```python
from build123d import *

# Parameters (mm, degrees)
SKETCH1_R           = 0.425
SKETCH1_R_2         = 0.8
BOSS_EXTRUDE1_DEPTH = 1.6


with BuildPart() as part:
    # Sketch1 → Boss-Extrude1 (new body)
    with BuildSketch(Plane(origin=(0, 0, -0.0125), x_dir=(-1, 0, 0), z_dir=(0, 0, -1))):
        with BuildLine():
            Line((47.8, -40.8), (49.3, -40.8))
            Line((49.3, -40.8), (49.3, 39.2))
            Line((49.3, 39.2), (43.2, 45.3))
            Line((43.2, 45.3), (35.500000017, 45.3))
            Line((35.500000017, 45.3), (35.500000017, 43.8))
            ThreePointArc((35.500000017, 43.8), (35.207106799, 43.092893219), (34.500000017, 42.8))
            Line((34.500000017, 42.8), (4.500000014, 42.8))
            ThreePointArc((4.500000014, 42.8), (3.792893232, 43.092893219), (3.500000014, 43.8))
            Line((3.500000014, 43.8), (3.500000014, 45.3))
            Line((3.500000014, 45.3), (-43.2, 45.3))
            Line((-43.2, 45.3), (-49.3, 39.2))
            Line((-49.3, 39.2), (-49.3, -40.4))
            Line((-49.3, -40.4), (-47.8, -40.4))
            ThreePointArc((-47.8, -40.4), (-47.092893219, -40.692893219), (-46.8, -41.4))
            Line((-46.8, -41.4), (-46.8, -46))
            ThreePointArc((-46.8, -46), (-46.507106781, -46.707106781), (-45.8, -47))
            Line((-45.8, -47), (-36.3, -47))
            ThreePointArc((-36.3, -47), (-35.592893219, -47.292893219), (-35.3, -48))
            Line((-35.3, -48), (-35.3, -50))
            Line((-35.3, -50), (35.3, -50))
            Line((35.3, -50), (35.3, -48))
            ThreePointArc((35.3, -48), (35.592893219, -47.292893219), (36.3, -47))
            Line((36.3, -47), (45.8, -47))
            ThreePointArc((45.8, -47), (46.507106781, -46.707106781), (46.8, -46))
            Line((46.8, -46), (46.8, -41.8))
            ThreePointArc((46.8, -41.8), (47.092893219, -41.092893219), (47.8, -40.8))
        make_face()
        with Locations(Location((-13.87, 38.33, 0), (0, 0, 180))):
            Circle(SKETCH1_R, mode=Mode.SUBTRACT)
        with Locations(Location((-22.54, 39.6, 0), (0, 0, 180))):
            Circle(SKETCH1_R, mode=Mode.SUBTRACT)
        with Locations(Location((-23.81, 40.87, 0), (0, 0, 180))):
            Circle(SKETCH1_R, mode=Mode.SUBTRACT)
        with Locations(Location((-21.27, 40.87, 0), (0, 0, 180))):
            Circle(SKETCH1_R, mode=Mode.SUBTRACT)
        with Locations(Location((-13.87, 40.87, 0), (0, 0, 180))):
            Circle(SKETCH1_R, mode=Mode.SUBTRACT)
        with Locations(Location((-31.21, 40.87, 0), (0, 0, 180))):
            Circle(SKETCH1_R, mode=Mode.SUBTRACT)
        with Locations(Location((-16.41, 40.87, 0), (0, 0, 180))):
            Circle(SKETCH1_R, mode=Mode.SUBTRACT)
        with Locations(Location((-15.14, 39.6, 0), (0, 0, 180))):
            Circle(SKETCH1_R, mode=Mode.SUBTRACT)
        with Locations(Location((-29.94, 39.6, 0), (0, 0, 180))):
            Circle(SKETCH1_R, mode=Mode.SUBTRACT)
        with Locations(Location((-28.67, 40.87, 0), (0, 0, 180))):
            Circle(SKETCH1_R, mode=Mode.SUBTRACT)
        with Locations(Location((-28.67, 38.33, 0), (0, 0, 180))):
            Circle(SKETCH1_R, mode=Mode.SUBTRACT)
        with Locations(Location((-16.41, 38.33, 0), (0, 0, 180))):
            Circle(SKETCH1_R, mode=Mode.SUBTRACT)
        with Locations(Location((-21.27, 38.33, 0), (0, 0, 180))):
            Circle(SKETCH1_R, mode=Mode.SUBTRACT)
        with Locations(Location((-23.81, 38.33, 0), (0, 0, 180))):
            Circle(SKETCH1_R, mode=Mode.SUBTRACT)
        with Locations(Location((-31.21, 38.33, 0), (0, 0, 180))):
            Circle(SKETCH1_R, mode=Mode.SUBTRACT)
        with Locations((33.775, 38.54)):
            Circle(SKETCH1_R_2, mode=Mode.SUBTRACT)
        with Locations((5.225, 38.54)):
            Circle(SKETCH1_R_2, mode=Mode.SUBTRACT)
    extrude(amount=-BOSS_EXTRUDE1_DEPTH)


solid = part.part
```
The model under review builds one solid part; all positions refer to its coordinate system, in mm. Round coordinates to 2 decimals unless told otherwise and drop trailing zeros. Order: outer loops, then holes, each group sorted by start corner. A loop starts at its lowest first (then second) coordinate and runs counter-clockwise, first axis right, second up.
Item 1: To check wall thickness, follow probe 1 along Y at (x, z) = (21.27, 0.3) (3 decimals); probe 2 along Y at (x, z) = (15.14, 1) (3 decimals); probe 3 along Y at (x, z) = (-16, 0.5). State the ranges of each line that lie inside material, in increasing order.
Working result:
probe 1: y = -50 to 37.905, 38.755 to 40.445, 41.295 to 45.3
probe 2: y = -50 to 39.175, 40.025 to 45.3
probe 3: y = -50 to 42.8
Item 2: For pin 1 (0.5 mm diameter, centred on y = -48.5, z = 1, fed in from -X); pin 2 (0.5 mm diameter, centred on y = -44, z = 0.5, fed in from +X); pin 3 (0.8 mm diameter, centred on x = 48.5, z = 0.5, fed in from -Y); pin 4 (1 mm diameter, centred on x = -33.775, y = 38.54, fed in from -Z), all flat-tipped, find the tip position at first contact; note any pin that passes through.
Working result:
pin 1: stops at x = -35.3
pin 2: stops at x = 46.8
pin 3: stops at y = -40.4
pin 4: passes through
Item 3: Add section A-A, the plane z = 0.7. Count the separate pieces of the cut face and the enclosed holes in it, and give its area (3 significant figures).
Working result:
separate pieces: 1
enclosed holes: 17
area: 9,150 mm2
Item 4: Add section B-B, the plane x = -9. State the section outline as (y, z) points.
Working result:
outline: (-50, -0.01) - (42.8, -0.01) - (42.8, 1.59) - (-50, 1.59) - close
